Design review of the part built by this model. Coordinates are the model's own, in mm. Face numbers are marked on the shaded views. A direction names the side the tool comes from. Coordinates: 2 decimals unless noted, no trailing zeros. Write each loop counter-clockwise with the first axis right and the second up, starting at its lowest first coordinate (ties: lowest second). Pieces come first, ordered by that corner, then holes. Notation, with made-up numbers: (4, -23.5) -> (8, -23.5) arc R20 ccw to (8, -15.5) -> close; hole circle Ø1 at (0.25, 9). An arc over 180 degrees is marked (long way). Answer in a Markdown table with one row per item. Add a question column.
Item 1: Take a section at C-C, the plane y = -1.75. Write out the cut boundary in (x, z).
Item 2: Take a section at B-B, the plane x = 0. Write out the cut boundary in (y, z), and give its area (3 significant figures).
Item 3: Clearance check with flat-ended pins moving along their axes: P1, Ø0.9, axis at y = -3.5, z = 17, coming from the +X side; P2, Ø3, axis at y = 5.5, z = 6, coming from the +X side; P3, Ø3, axis at y = 4.5, z = 6, coming from the +X side; P4, Ø3, axis at x = 0, z = 0, coming from the +Y side. State where each tip first meets the part, or that it passes through.
Item 4: To check wall thickness, follow line 1 (Y direction, x = -3, z = 6); line 2 (X direction, y = 6.5, z = 4.5); line 3 (Z direction, x = -0.25, y = 5.25). State the ranges of each line that lie inside material, in increasing order.
Item 5: Draft analysis for pull direction Y (two halves, no side actions). For the marked faces 6, 7 and 8, state which applies: released by +Y, released by -Y, zero draft, split by the parting line, or undercut.
Item 6: Take a section at D-D, the plane z = -0.75. Write out the cut boundary in (x, y).
Item 7: For the marked faces 1, 2, 3, 4 and 5, list the 3-axis set-ups (+Z, -Z, +X, -X, +Y, -Y) from which the entire face can be reached by the end or side of a thin tool; tool diameter is ignored.
Item 8: Take a section at A-A, the plane y = 4.5. Write out the cut boundary in (x, z).
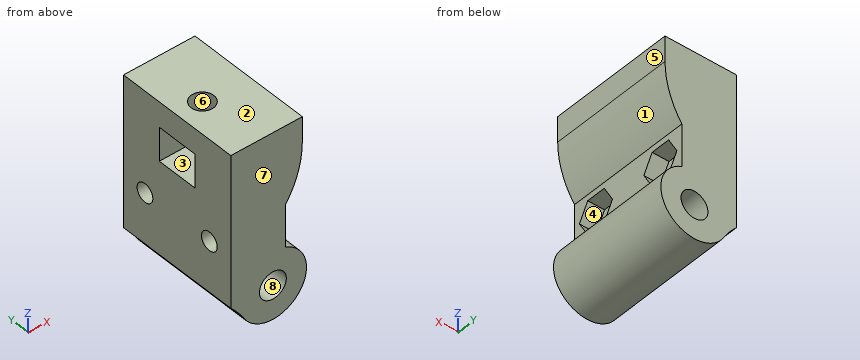
from build123d import *

# Parameters (mm, degrees)
SKETCH_1_R               = 1.6
EXTRUDE_1_DEPTH          = 7.5
CUT_EXTRUDE_1_DEPTH      = 21.554804791
CUT_EXTRUDE_1_DEPTH_BACK = 21.554804791
SKETCH_3_R               = 1.1
FILLET_1_R               = 10
SKETCH_6_R               = 1.35
CUT_EXTRUDE_2_DEPTH      = 4
SKETCH_7_W               = 4
SKETCH_7_H               = 5
CUT_EXTRUDE_3_DEPTH      = 6
CUT_EXTRUDE_4_DEPTH      = 21.554804791
CUT_EXTRUDE_4_DEPTH_BACK = 2


with BuildPart() as part:
    # 草图1 → 凸台-拉伸1 (new, symmetric)
    with BuildSketch(Plane(origin=(0, 0, 0), x_dir=(1, 0, 0), z_dir=(0, 1, 0))):
        with BuildLine():
            Line((-5, -18), (3.5, -18))
            Line((3.5, -18), (3.5, -15))
            ThreePointArc((3.5, -15), (2.987970346, -11.698938991), (1.5, -8.708099244))
            Line((1.5, -8.708099244), (1.5, -3.708099244))
            ThreePointArc((1.5, -3.708099244), (2.236067977, 3.31662479), (-4, 0))
            Line((-4, 0), (-5, 0))
            Line((-5, 0), (-5, -18))
        make_face()
        with Locations(Location((0, 0, 0), (0, 0, 270))):
            Circle(SKETCH_1_R, mode=Mode.SUBTRACT)
    extrude(amount=EXTRUDE_1_DEPTH, both=True)

    # 草图3 → 切除-拉伸1 (cut, two sides: drawn at the far end of the back side and taken through both)
    with BuildSketch(Plane(origin=(1.5, 0, 0), x_dir=(0, 0, -1), z_dir=(1, 0, 0)).offset(-CUT_EXTRUDE_1_DEPTH_BACK)):
        with Locations((-6, 4.5)):
            Circle(SKETCH_3_R)
        with Locations(Location((-6, -4.5, 0), (0, 0, 180))):
            Circle(SKETCH_3_R)
    extrude(amount=CUT_EXTRUDE_1_DEPTH + CUT_EXTRUDE_1_DEPTH_BACK, mode=Mode.SUBTRACT)

    # 圆角1
    # the kernel refuses this fillet: 10 mm, written as the material it adds along each edge
    with BuildSketch(Plane(origin=(-4, 7.5, 0), x_dir=(-1, 0, 0), z_dir=(0, -1, 0))) as fillet_1_piece_1:
        with BuildLine():
            CenterArc((8.1, 7.042016757), FILLET_1_R, 210.198757023, 14.566327648)
            Line((-0.542857143, 2.012004788), (-0.715714286, 1.911404548))
            ThreePointArc((-0.715714286, 1.911404548), (-0.331193265, 0.989877337), (-0.2, 0))
            Line((-0.2, 0), (0, -0.2))
            ThreePointArc((0, -0.2), (0.5, -0.2), (0.858, -0.140840335))
            Line((0.858, -0.140840335), (1, 0))
        make_face()
    extrude(amount=15)

    # 草图6 → 切除-拉伸2 (cut)
    with BuildSketch(Plane.XY.offset(18)):
        with Locations((-2, 0)):
            Circle(SKETCH_6_R)
    extrude(amount=-CUT_EXTRUDE_2_DEPTH, mode=Mode.SUBTRACT)

    # 草图7 → 切除-拉伸3 (cut)
    with BuildSketch(Plane.ZY.offset(5)):
        with Locations((13, 0)):
            Rectangle(SKETCH_7_W, SKETCH_7_H)
    extrude(amount=-CUT_EXTRUDE_3_DEPTH, mode=Mode.SUBTRACT)

    # 草图8 → 切除-拉伸4 (cut, two sides: drawn at the far end of the back side and taken through both)
    with BuildSketch(Plane(origin=(1.5, 0, 0), x_dir=(0, 0, -1), z_dir=(1, 0, 0)).offset(-CUT_EXTRUDE_4_DEPTH_BACK)):
        Polygon((-8, 5.654700538), (-8, 3.345299462), (-6, 2.190598923), (-4, 3.345299462), (-4, 5.654700538), (-6, 6.809401077), align=None)
        Polygon((-6, -6.809401077), (-8, -5.654700538), (-8, -3.345299462), (-6, -2.190598923), (-4, -3.345299462), (-4, -5.654700538), align=None)
    extrude(amount=CUT_EXTRUDE_4_DEPTH + CUT_EXTRUDE_4_DEPTH_BACK, mode=Mode.SUBTRACT)


solid = part.part
Answers:
| question | item | result |
|---|---|---|
| 1 | outline | (-5, 0) arc R10 cw to (-3.46, -2.01) arc R4 ccw (long way) to (1.5, 3.71) -> (1.5, 8.71) arc R10.9 ccw to (3.5, 15) -> (3.5, 18) -> (-5, 18) -> (-5, 15) -> (1, 15) -> (1, 11) -> (-5, 11) -> close; hole circle Ø3.2 at (0, 0) |
| 2 | outline | (-7.5, -4) -> (7.5, -4) -> (7.5, -1.6) -> (-7.5, -1.6) -> close; (-7.5, 1.6) -> (7.5, 1.6) -> (7.5, 18) -> (-7.5, 18) -> close; hole (-6.81, 6) -> (-5.65, 4) -> (-3.35, 4) -> (-2.19, 6) -> (-3.35, 8) -> (-5.65, 8) -> close; hole (-2.5, 11) -> (2.5, 11) -> (2.5, 15) -> (-2.5, 15) -> close; hole (2.19, 6) -> (3.35, 4) -> (5.65, 4) -> (6.81, 6) -> (5.65, 8) -> (3.35, 8) -> close |
| 2 | area | 234 mm^2 |
| 3 | P1 | stops at x = 3.5 |
| 3 | P2 | stops at x = 1.5 |
| 3 | P3 | stops at x = -0.5 |
| 3 | P4 | passes through |
| 4 | line 1 | y = -7.5 to -5.6, -3.4 to 3.4, 5.6 to 7.5 |
| 4 | line 2 | x = -5 to 1.5 |
| 4 | line 3 | z = -3.99 to -1.58, 1.58 to 4, 8 to 18 |
| 5 | face 6 | undercut |
| 5 | face 7 | released by -Y |
| 5 | face 8 | zero draft |
| 6 | outline | (-4.33, -7.5) -> (-1.41, -7.5) -> (-1.41, 7.5) -> (-4.33, 7.5) -> close; (1.41, -7.5) -> (3.93, -7.5) -> (3.93, 7.5) -> (1.41, 7.5) -> close |
| 7 | face 1 | +X, +Y, -Y |
| 7 | face 2 | +Z, +X, -X, +Y, -Y |
| 7 | face 3 | -X |
| 7 | face 4 | +X |
| 7 | face 5 | +Z, +X, +Y, -Y |
| 8 | outline | (-5, 0) arc R10 cw to (-3.46, -2.01) arc R4 ccw (long way) to (1.5, 3.71) -> (1.5, 4) -> (-0.5, 4) -> (-0.5, 4.9) -> (-5, 4.9) -> close; (-5, 7.1) -> (-0.5, 7.1) -> (-0.5, 8) -> (1.5, 8) -> (1.5, 8.71) arc R10.9 ccw to (3.5, 15) -> (3.5, 18) -> (-5, 18) -> close; hole circle Ø3.2 at (0, 0) |
